Drawing for the job (mm, zero at the part's lowest x, y, z). A direction names the side the tool comes from. Round coordinates to 2 decimals unless told otherwise and drop trailing zeros. Put each result on its own line as item: value. Start each with the question number.
Item 1: Saw through at B-B on y = 8.75. State how many separate pieces and enclosed holes the cut face has, plus the area to 3 significant figures.
Item 2: Probe probe 1 along X at (y, z) = (8.75, 23); probe 2 along X at (y, z) = (6.25, 39) (1 decimal); probe 3 along X at (y, z) = (4, 30.5) (1 decimal). List the from-to ranges inside material, lowest first.
Item 3: Which spindle directions (+Z, -Z, +X, -X, +Y, -Y) get a long thin tool onto all of the face, cutting with end or side? Do the marked faces 4 and 5. Say none if no direction does.
Item 4: Mould opens along Z. For the marked faces 1, 2 and 3 say: pulls with the +Z half, pulls with the -Z half, needs draft (parallel to the pull), parting line crosses it, or undercut.
Item 5: Pin check, flat tips, straight feed: pin 1 Ø3 at (x, y) = (33, 4) entering from +Z (1 decimal); pin 2 Ø1.9 at (y, z) = (5, 27) entering from +X (1 decimal); pin 3 Ø3 at (x, z) = (38, 18.5) entering from -Y. Stop position of each tip, or through.
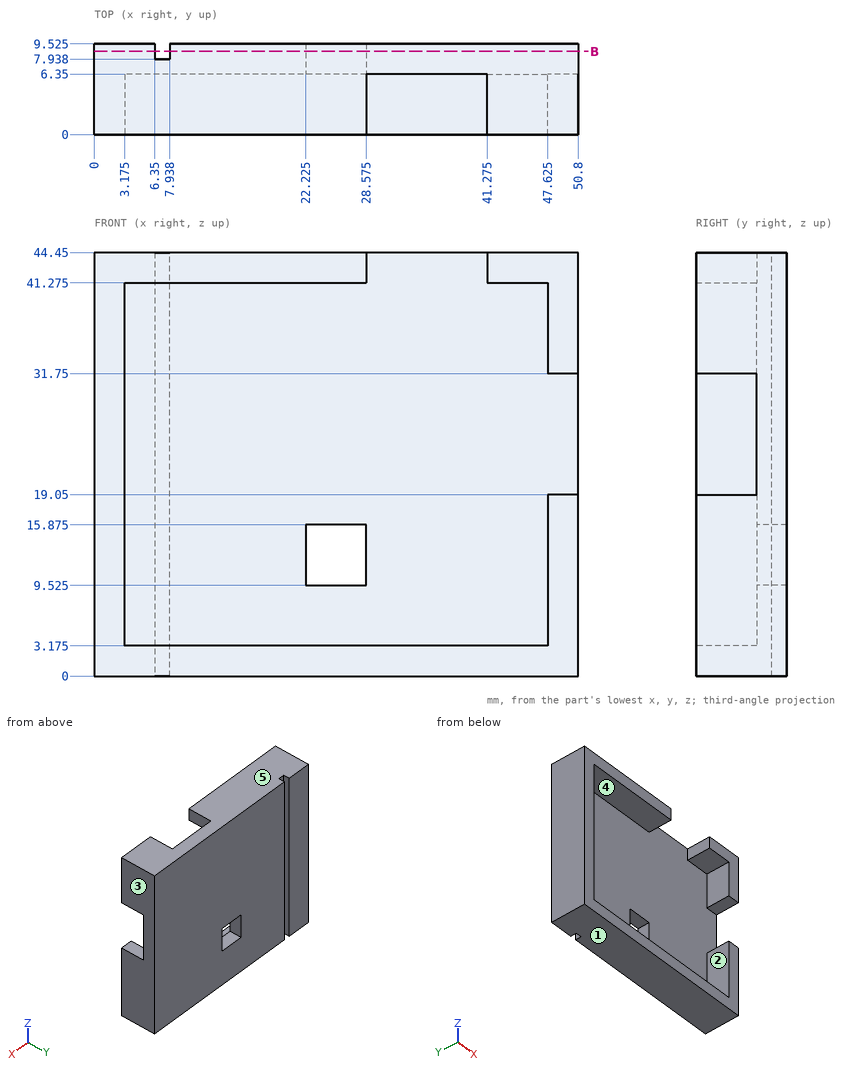
Results found:
1. separate pieces: 2
1. enclosed holes: 1
1. area: 2,150 mm²
2. probe 1: x = 0 to 6.35, 7.94 to 50.8
2. probe 2: x = 0 to 3.2, 47.6 to 50.8
2. probe 3: x = 0 to 3.2
3. face 4: -Y
3. face 5: +Z, +X, -X, +Y, -Y
4. face 1: pulls with the -Z half
4. face 2: undercut
4. face 3: needs draft
5. pin 1: stops at z = 3.2
5. pin 2: stops at x = 3.2
5. pin 3: stops at y = 6.35
